Geometry check sheet. Reference: the model listing, model coordinates, mm. A direction names the side the tool comes from. Give positions to 0.01 mm unless a question says otherwise; leave off trailing zeros. Write each loop counter-clockwise with the first axis right and the second up, starting at its lowest first coordinate (ties: lowest second). Pieces come first, ordered by that corner, then holes. Notation, with made-up numbers: (56.25, -39.75) - (108.25, -39.75) arc R16 ccw to (108.25, -17.75) - close; hole circle Ø8 at (83.5, 12). An arc over 180 degrees is marked (long way). One line per question, with ' | ' between items. Start each with the question number.
Q1. Set-up check for faces 4 (the face through (7, 3, 4)), 5 (the face through (3.5, 6, 2)), 6 (the face through (14, 1, 2)), 7 (the face through (0.5, 1, 2)): record each of +Z, -Z, +X, -X, +Y, -Y from which the full face is reachable in a straight line by a thin tool's end or side.
Q2. Thickness scan on L1, parallel to Y at x = 3.75, z = 2.6; L2, parallel to Y at x = 5, z = 0.35; L3, parallel to X at y = 0.75, z = 1.8. Record the ranges inside material, lowest first. Write a range as [from, to].
Q3. Section check C-C on z = 1.2. Record the boundary of the cut face in (x, y), and give its area (3 significant figures).
Q4. Gauge pin test, flat ends, axial feed: P1, Ø1.2, axis at x = 10.75, y = 3.5, coming from the -Z side (3 decimals); P2, Ø2, axis at x = 8.5, z = 1, coming from the +Y side; P3, Ø0.8, axis at y = 6.5, z = 2, coming from the +X side (3 decimals). Record the tip position at first contact, or that the pin passes through.
Q5. Section check D-D on y = 3.5. Record the boundary of the cut face in (x, z).
Q6. Release check for a two-part mould opening along Y. For faces 1 (the face through (0.301, 6.715, 1.972)), 2 (the face through (11, 6, 2)), 3 (the face through (3.155, 3.044, 1.972)) record: +Y half, -Y half, draft (parallel to the pull), parting line (faces both ways), or undercut.
Q7. Section check A-A on x = 10.75. Record the boundary of the cut face in (y, z), and give its area (3 significant figures).
Q8. Section check B-B on y = 5.75. Record the boundary of the cut face in (x, z).
```python
from build123d import *

# Parameters (mm, degrees)
F0_R     = 0.75
F1_DEPTH = 4


with BuildPart() as f1:
    # F0 (on Top) → F1 (new body)
    with BuildSketch(Plane.XY):
        with BuildLine():
            ThreePointArc((1, 7), (0.292893, 6.707107), (0, 6))
            ThreePointArc((0, 6), (1, 5), (2, 6))
            ThreePointArc((2, 6), (1.707107, 6.707107), (1, 7))
        make_face()
        with BuildLine():
            Line((0.5, 2.5), (0.5, 0))
            Line((0.5, 0), (14, 0))
            Line((14, 0), (14, 2.5))
            Line((14, 2.5), (14.5, 2.5))
            Line((14.5, 2.5), (14.5, 6))
            ThreePointArc((14.5, 6), (12.792893, 5.292893), (13.5, 7))
            Line((13.5, 7), (11, 7))
            Line((11, 7), (11, 5.5))
            Line((11, 5.5), (3.5, 5.5))
            Line((3.5, 5.5), (3.5, 7))
            Line((3.5, 7), (1, 7))
            ThreePointArc((1, 7), (1.707107, 6.707107), (2, 6))
            ThreePointArc((2, 6), (1, 5), (0, 6))
            Line((0, 6), (0, 2.5))
            Line((0, 2.5), (0.5, 2.5))
        make_face()
        with Locations((3.75, 3.5)):
            Circle(F0_R, mode=Mode.SUBTRACT)
        with Locations((10.75, 3.5)):
            Circle(F0_R, mode=Mode.SUBTRACT)
        with BuildLine():
            ThreePointArc((13.5, 7), (12.792893, 5.292893), (14.5, 6))
            ThreePointArc((14.5, 6), (14.207107, 6.707107), (13.5, 7))
        make_face()
    extrude(amount=F1_DEPTH)


solid = f1.part
```
Working result:
1) face 4: +Z, +X, -X, +Y, -Y | face 5: +Z, -Z, +Y | face 6: +Z, -Z, +X, -Y | face 7: +Z, -Z, -X, -Y
2) L1: y = [0, 2.75], [4.25, 5.5] | L2: y = [0, 5.5] | L3: x = [0.5, 14]
3) outline: (0, 2.5) - (0.5, 2.5) - (0.5, 0) - (14, 0) - (14, 2.5) - (14.5, 2.5) - (14.5, 6) arc R1 ccw to (13.5, 7) - (11, 7) - (11, 5.5) - (3.5, 5.5) - (3.5, 7) - (1, 7) arc R1 ccw to (0, 6) - close; hole circle Ø1.5 at (3.75, 3.5); hole circle Ø1.5 at (10.75, 3.5) | area: 83.8 mm2
4) P1: passes through | P2: stops at y = 5.5 | P3: stops at x = 14.495
5) outline: (0, 0) - (3, 0) - (3, 4) - (0, 4) - close; (4.5, 0) - (10, 0) - (10, 4) - (4.5, 4) - close; (11.5, 0) - (14.5, 0) - (14.5, 4) - (11.5, 4) - close
6) face 1: +Y half | face 2: draft | face 3: undercut
7) outline: (0, 0) - (2.75, 0) - (2.75, 4) - (0, 4) - close; (4.25, 0) - (5.5, 0) - (5.5, 4) - (4.25, 4) - close | area: 16.0 mm2
8) outline: (0, 0) - (3.5, 0) - (3.5, 4) - (0, 4) - close; (11, 0) - (14.5, 0) - (14.5, 4) - (11, 4) - close
